Input: part model. Units: mm. Frame: model coordinates. A direction names the side the tool comes from. Give positions to 0.01 mm unless a question says otherwise; leave off trailing zeros. Write each loop counter-clockwise with the first axis right and the second up, starting at its lowest first coordinate (ties: lowest second). Pieces come first, ordered by that corner, then holes. Notation, with made-up numbers: (21, 85.25) - (55, 85.25) arc R16 ccw to (55, 109.25) - close; hole circle Ø8 at (-36, -29). An arc over 180 degrees is marked (long way). Answer as CSV lines item,"result".
```python
from build123d import *

# Parameters (mm, degrees)
BOSS_EXTRUDE1_DEPTH             = 50
CUT_EXTRUDE1_REACH              = 23.5
SKETCH3_R                       = 2.5
CBORE_FOR_M3_SBHCS1_D           = 3.4
CBORE_FOR_M3_SBHCS1_CBORE_D     = 6.7
CBORE_FOR_M3_SBHCS1_CBORE_DEPTH = 1.65


with BuildPart() as part:
    # Sketch2 → Boss-Extrude1 (new body)
    with BuildSketch(Plane.XY):
        Polygon((-15.713485752, 63.637116303), (-18.483485752, 60.867117128), (-15.713485752, 58.097116303), (-1.213485752, 58.097116303), (-1.213485752, 51.097116303), (-22.713485752, 51.097116303), (-22.713485752, 65.637116303), (-15.713485752, 65.637116303), align=None)
    extrude(amount=BOSS_EXTRUDE1_DEPTH)

    # Sketch3 → Cut-Extrude1 (cut, up to next)
    with BuildSketch(Plane.ZY.offset(22.713485752), mode=Mode.PRIVATE) as cut_extrude1_sk1:
        with Locations((17, 55.097116303)):
            Circle(SKETCH3_R)
    cut_extrude1_tool1 = extrude(cut_extrude1_sk1.sketch, amount=-CUT_EXTRUDE1_REACH, mode=Mode.PRIVATE) & part.part
    add(cut_extrude1_tool1.solids().sort_by_distance((-22.713486, 55.097116, 17))[0], mode=Mode.SUBTRACT)
    # Sketch3 → Cut-Extrude1 (cut, up to next)
    with BuildSketch(Plane.ZY.offset(22.713485752), mode=Mode.PRIVATE) as cut_extrude1_sk2:
        with Locations((33, 55.097116303)):
            Circle(SKETCH3_R)
    cut_extrude1_tool2 = extrude(cut_extrude1_sk2.sketch, amount=-CUT_EXTRUDE1_REACH, mode=Mode.PRIVATE) & part.part
    add(cut_extrude1_tool2.solids().sort_by_distance((-22.713486, 55.097116, 33))[0], mode=Mode.SUBTRACT)

    # CBORE for M3 SBHCS1 (through all)
    with Locations(Plane(origin=(0, 58.097116303, 0), x_dir=(1, 0, 0), z_dir=(0, 1, 0))):
        with Locations((-9.219799779, -40), (-8.943485752, -10)):
            CounterBoreHole(CBORE_FOR_M3_SBHCS1_D / 2, CBORE_FOR_M3_SBHCS1_CBORE_D / 2, CBORE_FOR_M3_SBHCS1_CBORE_DEPTH)


solid = part.part
```
Item 1: Mould query, pull axis Z, two halves, no side actions, for faces 1 (the face through (-19, 65.637, 25)), 2 (the face through (-10, 53.73, 41.51)), 3 (the face through (-12.114, 55.207, 14.502)), 4 (the face through (-14, 57, 0)). Classes: +Z half, -Z half, draft (parallel to the pull), parting line (faces both ways), or undercut.
The answers:
face 1,"draft"
face 2,"undercut"
face 3,"undercut"
face 4,"-Z half"
Item 2: Contact query for flat-ended pins moving along their axis: pin 1 (1.6 mm diameter, centred on y = 64.5, z = 33.5, fed in from +X); pin 2 (7.5 mm diameter, centred on x = -8.94, z = 10, fed in from +Y); pin 3 (3.5 mm diameter, centred on x = -9, z = 39.5, fed in from +Y). Output: stop coordinate, or through.
The answers:
pin 1,"x = -15.71"
pin 2,"y = 58.1"
pin 3,"y = 56.45"
Item 3: Ray query, line 1 (Z direction, x = -14.25, y = 55); line 2 (X direction, y = 54.2, z = 40); line 3 (X direction, y = 57.1, z = 10). Return the intervals inside material, ascending. Write a range as from..to.
The answers:
line 1,"0..14.5, 19.5..30.5, 35.5..50"
line 2,"-22.71..-10.92, -7.52..-1.21"
line 3,"-22.71..-12.29, -5.59..-1.21"
Item 4: Reachability of faces 5 (the face through (-1.213, 55, 25)), 6 (the face through (-14, 57, 50)), 7 (the face through (-17.08, 62.27, 24.65)), 8 (the face through (-9, 58.097, 25)), 9 (the face through (-5.849, 57.284, 11.283)) from +Z, -Z, +X, -X, +Y, -Y: full face, straight path, thin tool, end or side. Return the list, or none.
The answers:
face 5,"+Z, -Z, +X, +Y, -Y"
face 6,"+Z, +X, -X, +Y, -Y"
face 7,"+Z, -Z, +X"
face 8,"+Z, -Z, +X, +Y"
face 9,"+Y"
Item 5: Cut plane B-B on y = 54.5. Return the cut outline in (x, z), plus the area to 3 significant figures.
The answers:
outline,"(-22.71, 0) - (-1.21, 0) - (-1.21, 14.57) - (-22.71, 14.57) - close; (-22.71, 19.43) - (-1.21, 19.43) - (-1.21, 30.57) - (-22.71, 30.57) - close; (-22.71, 35.43) - (-1.21, 35.43) - (-1.21, 50) - (-22.71, 50) - close; hole circle Ø3.4 at (-9.22, 40); hole circle Ø3.4 at (-8.94, 10)"
area,"848 mm²"
Item 6: Cut plane A-A on z = 33. Return the cut outline in (x, y).
The answers:
outline,"(-22.71, 51.1) - (-1.21, 51.1) - (-1.21, 52.6) - (-22.71, 52.6) - close; (-22.71, 57.6) - (-1.21, 57.6) - (-1.21, 58.1) - (-15.71, 58.1) - (-18.48, 60.87) - (-15.71, 63.64) - (-15.71, 65.64) - (-22.71, 65.64) - close"
Item 7: Cut plane D-D on z = 40. Return the cut outline in (x, y).
The answers:
outline,"(-22.71, 51.1) - (-10.92, 51.1) - (-10.92, 56.45) - (-12.57, 56.45) - (-12.57, 58.1) - (-15.71, 58.1) - (-18.48, 60.87) - (-15.71, 63.64) - (-15.71, 65.64) - (-22.71, 65.64) - close; (-7.52, 51.1) - (-1.21, 51.1) - (-1.21, 58.1) - (-5.87, 58.1) - (-5.87, 56.45) - (-7.52, 56.45) - close"
Item 8: Cut plane C-C on x = -16.75. Return the cut outline in (y, z), plus the area to 3 significant figures.
The answers:
outline,"(51.1, 0) - (59.13, 0) - (59.13, 50) - (51.1, 50) - close; (62.6, 0) - (65.64, 0) - (65.64, 50) - (62.6, 50) - close; hole circle Ø5 at (55.1, 17); hole circle Ø5 at (55.1, 33)"
area,"514 mm²"
